Model file for the job. Use its own axes, mm. Face numbers are marked on the shaded views. A direction names the side the tool comes from. Give positions to 0.01 mm unless a question says otherwise; leave off trailing zeros. Write each loop counter-clockwise with the first axis right and the second up, starting at its lowest first coordinate (ties: lowest second). Pieces come first, ordered by that corner, then holes. Notation, with made-up numbers: (36.5, -3.75) - (93.5, -3.75) arc R19 cw to (93.5, 6.25) - close; hole circle Ø1 at (-22.75, 20). An arc over 180 degrees is marked (long way). Use a Markdown table: item, result. Add a question column.
```python
from build123d import *

# Parameters (mm, degrees)
F0_R     = 6.25
F0_W     = 15
F0_H     = 20
F0_W_2   = 93.98
F0_W_3   = 3.02
F0_W_4   = 3
F1_DEPTH = 22
F2_DEPTH = 30.48
F3_DEPTH = 18
F4_SIZE  = 4
F5_R     = 5


with BuildPart() as f1:
    # F0 (on Top) → F1 (new body)
    with BuildSketch(Plane.XY):
        Polygon((15, 10), (15, 50), (-15, 50), (-15, -50), (15, -50), (15, -10), (0, -10), (0, 10), align=None)
        with Locations((0, -35)):
            Circle(F0_R, mode=Mode.SUBTRACT)
        with Locations((0, 35)):
            Circle(F0_R, mode=Mode.SUBTRACT)
        with Locations((7.5, 0)):
            Rectangle(F0_W, F0_H)
        with Locations((68.01, 0)):
            Rectangle(F0_W_2, F0_H)
        with Locations((0, -35)):
            Circle(F0_R)
        with Locations((0, 35)):
            Circle(F0_R)
        with Locations((16.51, 0)):
            Rectangle(F0_W_3, F0_H)
        with Locations((19.52, 0)):
            Rectangle(F0_W_4, F0_H)
    extrude(amount=F1_DEPTH)

    # F0 (on Top) → F2 (join)
    with BuildSketch(Plane.XY):
        with Locations((116.5, 0)):
            Rectangle(F0_W_4, F0_H)
        with Locations((19.52, 0)):
            Rectangle(F0_W_4, F0_H)
    extrude(amount=F2_DEPTH)

    # F0 (on Top) → F3 (cut)
    with BuildSketch(Plane.XY):
        with Locations((0, -35)):
            Circle(F0_R)
        with Locations((0, 35)):
            Circle(F0_R)
    extrude(amount=F3_DEPTH, mode=Mode.SUBTRACT)

    # F4
    f4_edges = [f1.edges().sort_by_distance(p)[0] for p in [
        (-6.25, -35, 18),
        (-6.25, 35, 18),
    ]]
    chamfer(f4_edges, length=F4_SIZE)

    # F5
    f5_edges = [f1.edges().sort_by_distance(p)[0] for p in [
        (68.01, -10, 22),
        (68.01, 10, 22),
        (116.5, -10, 30.48),
        (116.5, 10, 30.48),
        (15, -30, 22),
        (15, 30, 22),
        (-15, 0, 22),
        (0, -50, 22),
        (0, 50, 22),
        (19.52, -10, 30.48),
        (19.52, 10, 30.48),
        (16.51, 10, 22),
        (16.51, -10, 22),
    ]]
    fillet(f5_edges, radius=F5_R)


solid = f1.part
```
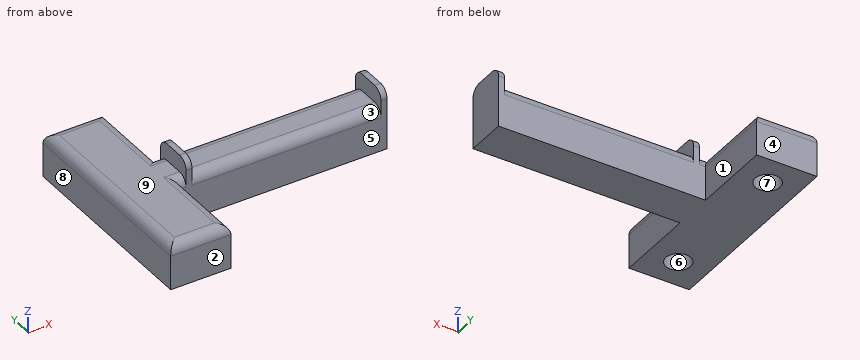
(1) Two-plate mould, pull along X, no slides. Class the marked faces 6, 7, 8 and 9: +X half, -X half, draft (parallel to the pull), parting line (faces both ways), or undercut.
(2) Probe probe 1 along Y at (x, z) = (0, 11.25); probe 2 along Y at (x, z) = (60.5, 8); probe 3 along X at (y, z) = (-21.5, 2.5). List the from-to ranges inside material, lowest first. Write a range as [from, to].
(3) Band-saw the part on D-D (x = 58). Write the cut outline in (y, z), then the cut area to 3 significant figures.
(4) Band-saw the part on B-B (x = 0). Write the cut outline in (y, z), then the cut area to 3 significant figures.
(5) Flat gauge pins, fed straight in: pin 1 (4 mm diameter, centred on y = 2.5, z = 26, fed in from -X); pin 2 (6 mm diameter, centred on x = 0.5, z = 21.5, fed in from +Y); pin 3 (2 mm diameter, centred on x = 1, y = -34.5, fed in from -Z); pin 4 (10 mm diameter, centred on x = 14.5, y = 29.5, fed in from -Z). Where does each tip first touch, or does it go through?
(6) Which spindle directions (+Z, -Z, +X, -X, +Y, -Y) get a long thin tool onto all of the face, cutting with end or side? Do the marked faces 1, 2, 3, 4 and 5. Say none if no direction does.
(7) Band-saw the part on A-A (z = 11.5). Write the cut outline in (x, y).
(8) Band-saw the part on C-C (y = -35). Write the cut outline in (x, z).
Model answer:
| question | item | result |
|---|---|---|
| 1 | face 6 | undercut |
| 1 | face 7 | undercut |
| 1 | face 8 | -X half |
| 1 | face 9 | draft |
| 2 | probe 1 | y = [-50, -41.25], [-28.75, 28.75], [41.25, 50] |
| 2 | probe 2 | y = [-10, 10] |
| 2 | probe 3 | x = [-15, 15] |
| 3 | outline | (-10, 0) - (10, 0) - (10, 17) arc R5 ccw to (5, 22) - (-5, 22) arc R5 ccw to (-10, 17) - close |
| 3 | area | 429 mm^2 |
| 4 | outline | (-50, 0) - (-41.25, 0) - (-41.25, 14) - (-37.25, 18) - (-32.75, 18) - (-28.75, 14) - (-28.75, 0) - (28.75, 0) - (28.75, 14) - (32.75, 18) - (37.25, 18) - (41.25, 14) - (41.25, 0) - (50, 0) - (50, 17) arc R5 ccw to (45, 22) - (-45, 22) arc R5 ccw to (-50, 17) - close |
| 4 | area | 1,770 mm^2 |
| 5 | pin 1 | stops at x = 18.02 |
| 5 | pin 2 | stops at y = 49.77 |
| 5 | pin 3 | stops at z = 18 |
| 5 | pin 4 | stops at z = 0 |
| 6 | face 1 | +Z, -Z, +X, +Y |
| 6 | face 2 | +Z, -Z, +X, -X, -Y |
| 6 | face 3 | +Z, -Y |
| 6 | face 4 | +Z, -Z, +X, -X, +Y |
| 6 | face 5 | +Z, -Z, +X, -Y |
| 7 | outline | (-15, -50) - (15, -50) - (15, -10) - (118, -10) - (118, 10) - (15, 10) - (15, 50) - (-15, 50) - close; hole circle Ø12.5 at (0, -35); hole circle Ø12.5 at (0, 35) |
| 8 | outline | (-15, 0) - (-6.25, 0) - (-6.25, 14) - (-2.25, 18) - (2.25, 18) - (6.25, 14) - (6.25, 0) - (15, 0) - (15, 17) arc R5 ccw to (10, 22) - (-10, 22) arc R5 ccw to (-15, 17) - close |
